Check sheet for the modelled part. Datum: model origin and axes. Units: mm. A direction names the side the tool comes from. Give positions to 0.01 mm unless a question says otherwise; leave off trailing zeros. Loops run counter-clockwise (first coordinate to the right, second up) from the corner with the lowest first, then second, coordinate; pieces in that order, holes last. Notation, with made-up numbers: (62.5, 71.5) -> (118.5, 71.5) arc R24 ccw to (118.5, 84.5) -> close; hole circle Ø8 at (5.25, 33.5). An arc over 180 degrees is marked (long way). Answer as CSV lines item,"result". Start each with the question number.
(1) Material ranges on line 1 (Y direction, x = 58.42, z = 10.75); line 2 (Z direction, x = 63, y = 10) (3 decimals); line 3 (X direction, y = 6, z = 50), recorded low to high. Write a range as from..to.
(2) Section check C-C on y = -4. Enter the section's corners in (x, z) (3 decimals).
(3) Release check for a two-part mould opening along X. For faces 4 (the face through (-48, 6, 79.375)), 5 (the face through (-54.415, 7.764, 53.661)), 6 (the face through (-72.38, -44.13, 7.76)) record: pulls with the +X half, pulls with the -X half, needs draft (parallel to the pull), parting line crosses it, or undercut.
(4) Section check A-A on x = 58.42. Enter the section's corners in (y, z) (3 decimals), plus the area to 3 significant figures.
(5) Access from +Z, -Z, +X, -X, +Y, -Y to the whole of each face (thin tool, end or side, straight path). Record for faces 1 (the face through (67.2, -18.2, 15.748)), 2 (the face through (-68, -18, 15.748)), 3 (the face through (-76.2, -18, 8)).
(6) Section check D-D on y = -18. Enter the section's corners in (x, z) (3 decimals).
(7) Gauge pin test, flat ends, axial feed: pin 1 Ø11.5 at (x, z) = (63.5, 50.8) entering from +Y; pin 2 Ø14.5 at (y, z) = (-33, 39) entering from +X; pin 3 Ø4.5 at (y, z) = (-16.5, 5.5) entering from -X; pin 4 Ø8 at (y, z) = (-9.5, 10.5) entering from +X. Record the tip position at first contact, or that the pin passes through.
(8) Section check B-B on z = 26. Enter the section's corners in (x, y), plus the area to 3 significant figures.
Autodesk Inventor part; units mm, degrees
ref_plane "YZ Plane" through (0, 0, 0) normal (1, 0, 0) x (0, 1, 0)
ref_plane "XZ Plane" through (0, 0, 0) normal (0, 1, 0) x (-1, 0, 0)
ref_plane "XY Plane" through (0, 0, 0) normal (0, 0, 1) x (1, 0, 0)
sketch "Sketch1" plane through (0, 0, 0) normal (0, 0, 1) x (1, 0, 0)
  line L0 (-95.25, 15.748) -> (95.25, 15.748)
  line L1 (95.25, 15.748) -> (95.25, 0)
  line L2 (95.25, 0) -> (-95.25, 0)
  line L3 (-95.25, 0) -> (-95.25, 15.748)
  line L4 (-76.2, 0) -> (76.2, 0)
  line L5 (76.2, 0) -> (76.2, -35.052)
  line L6 (63.5, -47.752) -> (-63.5, -47.752)
  line L7 (-76.2, -35.052) -> (-76.2, 0)
  arc A0 (-76.2, -35.052) -> (-63.5, -47.752) centre (-63.5, -35.052) ccw
  arc A1 (63.5, -47.752) -> (76.2, -35.052) centre (63.5, -35.052) ccw
  line L8 (-58.42, -22.352) -> (58.42, -22.352) construction
  line L9 (-58.42, -22.352) -> (58.42, -22.352) construction
  line L10 (0, -22.352) -> (0, -47.752) construction
  line L11 (-44.45, 15.748) -> (44.45, 15.748)
  line L12 (44.45, 15.748) -> (44.45, -47.752)
  line L13 (44.45, -47.752) -> (-44.45, -47.752)
  line L14 (-44.45, -47.752) -> (-44.45, 15.748)
  point P0 (0, 0)
  point P1 (0, 0)
  point P2 (0, 15.748)
  dimension "d0" = 190.5
  dimension "d1" = 15.748
  dimension "d4" = 63.5
  dimension "d5" = 152.4
  dimension "d6" = 12.7
  dimension "d7" = 12.7
  dimension "d8" = 116.84
  dimension "d9" = 0
  dimension "d10" = 25.4
  dimension "d11" = 63.5
  dimension "d12" = 88.9
extrude "Extrusion1" add sketch "Sketch1" along normal blind 79.375 contours L0 L14 L2 L3 | L0 L12 L2 L14 | L0 L1 L2 L12 | L2 L12 L6 L14
extrude "Extrusion2" add sketch "Sketch1" along normal blind 15.748 contours L14 L6 A0 L7 L2 | L2 L12 L6 L14 | L2 L5 A1 L6 L12
sketch "Sketch2" plane through (-44.45, -47.752, 79.375) normal (0, -1, 0) x (1, 0, 0)
  line L0 (139.7, 0) -> (-50.8, 0) construction
  circle A0 centre (44.45, 0) radius 28.575
  line L1 (-19.05, 0) -> (107.95, 0) construction
  line L2 (0, 0) -> (88.9, 0) construction
  line L3 (-19.05, 0) -> (-19.05, -28.575) construction
  line L4 (44.45, 0) -> (44.45, -8.2892) construction
  circle A1 centre (-19.05, -28.575) radius 9.525
  circle A2 centre (107.95, -28.575) radius 9.525
  point P0 (44.45, -79.375)
  dimension "d17" = 57.15
  dimension "d18" = 127
  dimension "d23" = 28.575
  dimension "d24" = 19.05
extrude "Extrusion3" cut sketch "Sketch2" against normal blind 63.5
hole "Hole1" at (-58.42, -22.352, 0) at (58.42, -22.352, 0) direction (0, 0, 1) diameter 19.05 end through all
properties part number "B"
Working result:
1,line 1,"y = -47.75..-31.88, -12.83..15.75"
1,line 2,"z = 0..41.288, 60.312..79.375"
1,line 3,"x = -95.25..-72.99, -54.01..54.01, 72.99..95.25"
2,outline,"(-76.2, 0) -> (76.2, 0) -> (76.2, 15.748) -> (44.45, 15.748) -> (44.45, 79.375) -> (28.575, 79.375) arc R28.575 cw to (-28.575, 79.375) -> (-44.45, 79.375) -> (-44.45, 15.748) -> (-76.2, 15.748) -> close"
3,face 4,"needs draft"
3,face 5,"undercut"
3,face 6,"pulls with the -X half"
4,outline,"(-47.752, 0) -> (-31.877, 0) -> (-31.877, 15.748) -> (-47.752, 15.748) -> close; (-12.827, 0) -> (15.748, 0) -> (15.748, 42.743) -> (0, 42.743) -> (0, 15.748) -> (-12.827, 15.748) -> close; (0, 58.857) -> (15.748, 58.857) -> (15.748, 79.375) -> (0, 79.375) -> close"
4,area,"1,450 mm^2"
5,face 1,"+Z, +X, -Y"
5,face 2,"+Z, -X, -Y"
5,face 3,"+Z, -Z, -X, -Y"
6,outline,"(-76.2, 0) -> (-66.893, 0) -> (-66.893, 15.748) -> (-76.2, 15.748) -> close; (-49.947, 0) -> (49.947, 0) -> (49.947, 15.748) -> (44.45, 15.748) -> (44.45, 79.375) -> (28.575, 79.375) arc R28.575 cw to (-28.575, 79.375) -> (-44.45, 79.375) -> (-44.45, 15.748) -> (-49.947, 15.748) -> close; (66.893, 0) -> (76.2, 0) -> (76.2, 15.748) -> (66.893, 15.748) -> close"
7,pin 1,"passes through"
7,pin 2,"stops at x = 44.45"
7,pin 3,"stops at x = -76.2"
7,pin 4,"stops at x = 76.2"
8,outline,"(-95.25, 0) -> (-44.45, 0) -> (-44.45, -47.75) -> (44.45, -47.75) -> (44.45, 0) -> (95.25, 0) -> (95.25, 15.75) -> (-95.25, 15.75) -> close"
8,area,"7,250 mm^2"
